```python
from build123d import *

# Parameters (mm, degrees)
SKETCH1_W             = 390
SKETCH1_H             = 90
BOSS_EXTRUDE1_DEPTH   = 3.175
SKETCH2_W             = 143
SKETCH2_H             = 63
CUT_EXTRUDE1_DEPTH    = 3.175
M4X0_7_TAPPED_HOLE1_D = 3.3
SKETCH6_W             = 22.475
SKETCH6_H             = 70
CUT_EXTRUDE2_DEPTH    = 3.175
M4_CLEARANCE_HOLE2_D  = 4.5


with BuildPart() as part:
    # Sketch1 → Boss-Extrude1 (new body)
    with BuildSketch(Plane(origin=(0, 0, 0), x_dir=(0, 0, -1), z_dir=(1, 0, 0))):
        Rectangle(SKETCH1_W, SKETCH1_H)
    extrude(amount=BOSS_EXTRUDE1_DEPTH)

    # Sketch2 → Cut-Extrude1 (cut)
    with BuildSketch(Plane(origin=(3.175, 0, 0), x_dir=(0, 0, -1), z_dir=(1, 0, 0))):
        with Locations((72.675, 0)):
            Rectangle(SKETCH2_W, SKETCH2_H)
        with Locations((-103.825, 0)):
            Rectangle(SKETCH2_W, SKETCH2_H)
    extrude(amount=-CUT_EXTRUDE1_DEPTH, mode=Mode.SUBTRACT)

    # M4x0.7 Tapped Hole1 (through all)
    with Locations(Plane(origin=(3.175, 0, 0), x_dir=(0, 0, -1), z_dir=(1, 0, 0))):
        with Locations((-103.825, 0), (-28.075, 35.75), (-179.575, -35.75), (-179.575, 35.75), (-28.075, -35.75), (72.675, 0), (148.425, 35.75), (-3.075, -35.75), (-3.075, 35.75), (148.425, -35.75)):
            Hole(M4X0_7_TAPPED_HOLE1_D / 2)

    # Sketch6 → Cut-Extrude2 (cut)
    with BuildSketch(Plane(origin=(3.175, 0, 0), x_dir=(0, 0, -1), z_dir=(1, 0, 0))):
        with Locations((175.5875, 0)):
            Rectangle(SKETCH6_W, SKETCH6_H)
    extrude(amount=-CUT_EXTRUDE2_DEPTH, mode=Mode.SUBTRACT)

    # M4 Clearance Hole2 (through all)
    with Locations(Plane(origin=(3.175, 0, 0), x_dir=(0, 0, -1), z_dir=(1, 0, 0))):
        with Locations((-103.825, 0), (-19.825, 40), (-187.825, -40), (-187.825, 40), (-19.825, -40), (72.675, 0), (156.675, 40), (-11.325, -40), (-11.325, 40), (156.675, -40)):
            Hole(M4_CLEARANCE_HOLE2_D / 2)


solid = part.part
```
Geometry check sheet. Reference: the model listing, model coordinates, mm. Give positions to 0.01 mm unless a question says otherwise; leave off trailing zeros. Order: outer loops, then holes, each group sorted by start corner. A loop starts at its lowest first (then second) coordinate and runs counter-clockwise, first axis right, second up. Notation, with made-up numbers: (-1, -12) - (25, -12) arc R25 ccw to (25, 5) - close; hole circle Ø3 at (68.5, 42). An arc over 180 degrees is marked (long way). Answer in a Markdown table with one row per item. Add a question column.
Q1. Cross-section at A-A, the plane z = 105. Enter the section's corners in (x, y) (3 decimals).
Q2. Material ranges on probe 1 along Z at (x, y) = (2.75, 16) (3 decimals); probe 2 along Y at (x, z) = (1.05, 158); probe 3 along Y at (x, z) = (1.55, 11), recorded low to high. Write a range as from..to.
Q3. Cross-section at B-B, the plane x = 1.2. Count the separate pieces of the cut face and the enclosed holes in it, then the cut area to 3 significant figures.
Check values:
| question | item | result |
|---|---|---|
| 1 | outline | (0, -45) - (3.175, -45) - (3.175, -31.5) - (0, -31.5) - close; (0, 31.5) - (3.175, 31.5) - (3.175, 45) - (0, 45) - close |
| 2 | probe 1 | z = -195..-186.825, -164.35..-144.175, -1.175..32.325, 175.325..195 |
| 2 | probe 2 | y = -45..-31.5, 31.5..45 |
| 2 | probe 3 | y = -45..-42.23, -37.77..37.77, 42.23..45 |
| 3 | separate pieces | 1 |
| 3 | enclosed holes | 19 |
| 3 | area | 15,300 mm^2 |
